Autodesk Inventor part; units mm, degrees
ref_plane "YZ Plane" through (0, 0, 0) normal (1, 0, 0) x (0, 1, 0)
ref_plane "XZ Plane" through (0, 0, 0) normal (0, 1, 0) x (-1, 0, 0)
ref_plane "XY Plane" through (0, 0, 0) normal (0, 0, 1) x (1, 0, 0)
sketch "Sketch1" plane through (0, 0, 0) normal (0, 1, 0) x (-1, 0, 0)
  line L0 (-10.8149, 6.985) -> (6.4571, 6.985)
  line L1 (6.4571, 6.985) -> (6.4571, -6.985)
  line L2 (6.4571, -6.985) -> (-10.8149, -6.985)
  line L3 (-10.8149, -6.985) -> (-10.8149, 6.985)
  point P0 (0, 0)
  dimension "d0" = 13.97
  dimension "d1" = 17.272
  dimension "d2" = 6.985
extrude "Extrusion1" add sketch "Sketch1" along normal blind 9.144
sketch "Sketch3" plane through (10.8149, 0, 6.985) normal (1, 0, 0) x (0, 0, -1)
  line L0 (13.97, 0) -> (13.97, 9.144)
  line L1 (0, 0) -> (0, 9.144)
  circle A0 centre (3.4925, 4.572) radius 3.175
  circle A1 centre (10.4775, 4.572) radius 3.175
  point P0 (6.985, 0)
  dimension "d6" = 6.35
  dimension "d7" = 6.35
  dimension "d8" = 3.4925
  dimension "d9" = 3.4925
extrude "Extrusion2" cut sketch "Sketch3" against normal blind 4.572
properties part number "TE_2Pin"
Geometry: final body of the model. Coordinates: model frame, mm. A direction names the side the tool comes from. Give positions to 0.01 mm unless a question says otherwise; leave off trailing zeros. Write each loop counter-clockwise with the first axis right and the second up, starting at its lowest first coordinate (ties: lowest second). Pieces come first, ordered by that corner, then holes. Notation, with made-up numbers: (-9.75, 42) -> (9.25, 42) arc R12 ccw to (9.25, 54) -> close; hole circle Ø2 at (17, 83). An arc over 180 degrees is marked (long way). Answer in a Markdown table with one row per item.
(1) Section query B-B on y = 2. Return loops of the section in (x, z) (3 decimals).
Answers below:
| item | result |
|---|---|
| outline | (-6.457, -6.985) -> (10.815, -6.985) -> (10.815, -5.354) -> (6.243, -5.354) -> (6.243, -1.631) -> (10.815, -1.631) -> (10.815, 1.631) -> (6.243, 1.631) -> (6.243, 5.354) -> (10.815, 5.354) -> (10.815, 6.985) -> (-6.457, 6.985) -> close |
(2) Pin query (flat end, axial travel): pin 1 (3 mm diameter, centred on y = 5.5, z = -4, fed in from +X). Return the tip coordinate at first contact, or that it passes through.
Answers below:
| item | result |
|---|---|
| pin 1 | x = 6.24 |
(3) Section query C-C on x = 7.25. State how many separate pieces and enclosed holes the cut face has, then the cut area to 3 significant figures.
Answers below:
| item | result |
|---|---|
| separate pieces | 1 |
| enclosed holes | 2 |
| area | 64.4 mm^2 |
(4) Draft query along Y for faces 3 (the flat face through (2, 0, 0)), 4 (the flat face through (2, 9.144, 0)), 5 (the flat face through (2, 5, 6.985)), 6 (the cylindrical face through (8.56, 7.72, -3.08)). Return one class per face: +Y half, -Y half, draft (parallel to the pull), parting line (faces both ways), or undercut.
Answers below:
| item | result |
|---|---|
| face 3 | -Y half |
| face 4 | +Y half |
| face 5 | draft |
| face 6 | undercut |
(5) Section query A-A on z = 3.5. Return loops of the section in (x, y), then the cut area to 3 significant figures.
Answers below:
| item | result |
|---|---|
| outline | (-6.46, 0) -> (10.81, 0) -> (10.81, 1.4) -> (6.24, 1.4) -> (6.24, 7.75) -> (10.81, 7.75) -> (10.81, 9.14) -> (-6.46, 9.14) -> close |
| area | 129 mm^2 |
(6) Set-up query: faces 1 (the flat face through (2, 5, -6.985)), 2 (the flat face through (6.243, 5, -3)). Return all of +Z, -Z, +X, -X, +Y, -Y with unobstructed straight access to the full face (end or side cutting, diameter ignored); none if empty.
Answers below:
| item | result |
|---|---|
| face 1 | -Z, +X, -X, +Y, -Y |
| face 2 | +X |
(7) Ray query, line 1 along Y through (x, z) = (7.5, 3.5); line 2 along Z through (x, y) = (9.25, 3.75) (3 decimals); line 3 along Z through (x, y) = (7.5, 2.5) (3 decimals). Return the intervals inside material, ascending. Write a range as [from, to].
Answers below:
| item | result |
|---|---|
| line 1 | [0, 1.4], [7.75, 9.14] |
| line 2 | [-6.985, -6.559], [-0.426, 0.426], [6.559, 6.985] |
| line 3 | [-6.985, -5.898], [-1.087, 1.087], [5.898, 6.985] |
(8) Section query D-D on z = -2.75. Return loops of the section in (x, y).
Answers below:
| item | result |
|---|---|
| outline | (-6.46, 0) -> (10.81, 0) -> (10.81, 1.49) -> (6.24, 1.49) -> (6.24, 7.66) -> (10.81, 7.66) -> (10.81, 9.14) -> (-6.46, 9.14) -> close |
